Source: CAD feature listing. Evaluate the final solid. Frame: model axes, mm. Face numbers are marked on the shaded views. A direction names the side the tool comes from. Give positions to 0.01 mm unless a question says otherwise; leave off trailing zeros. Loops run counter-clockwise (first coordinate to the right, second up) from the corner with the lowest first, then second, coordinate; pieces in that order, holes last.
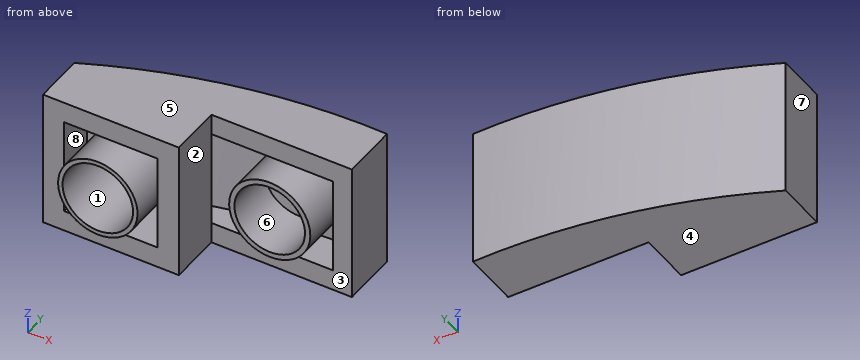
```python
from build123d import *

# Parameters (mm, degrees)
BOSS_EXTRUDE1_DEPTH      = 3.95
SHELL1_START             = -2.75
SHELL1_DEPTH             = 5.5
BOSS_EXTRUDE2_REACH      = 12.601
BOSS_EXTRUDE2_END_RADIUS = 32.700000868
BOSS_EXTRUDE2_START      = 1.2
SKETCH8_R                = 2.3
SKETCH8_R_2              = 2
BOSS_EXTRUDE3_REACH      = 13.983
BOSS_EXTRUDE3_END_RADIUS = 32.700000868
BOSS_EXTRUDE3_START      = 1.2
SKETCH9_R                = 2.25
SKETCH9_R_2              = 2
CUT_EXTRUDE5_DEPTH       = 13.479454835


# Read off the part's stored shape, not the designer's step: Shell1
with BuildPart() as part:
    # Sketch1 → Boss-Extrude1 (new, symmetric)
    with BuildSketch(Plane.XY):
        with BuildLine():
            Line((-7.9, -0.625209461), (-7.9, 2.229657062))
            ThreePointArc((-7.9, 2.229657062), (-0.19997769, 4.839494926), (7.9, 5.540892579))
            Line((7.9, 5.540892579), (7.9, 2.340892579))
            Line((7.9, 2.340892579), (-0.19997769, 2.340892579))
            Line((-0.19997769, 2.340892579), (-0.19997769, -0.625209461))
            Line((-0.19997769, -0.625209461), (-7.9, -0.625209461))
        make_face()
    extrude(amount=BOSS_EXTRUDE1_DEPTH, both=True)

    # Shell1 outline → Shell1 (cut)
    with BuildSketch(Plane.XY.offset(SHELL1_START)):
        with BuildLine():
            Line((-1.39997769, 2.340892579), (6.7, 2.340892579))
            Line((6.7, 2.340892579), (6.7, 4.360243445))
            ThreePointArc((6.7, 4.360243445), (-0.153454716, 3.622525068), (-6.7, 1.464559639))
            Line((-6.7, 1.464559639), (-6.7, -0.625209461))
            Line((-6.7, -0.625209461), (-1.39997769, -0.625209461))
            Line((-1.39997769, -0.625209461), (-1.39997769, 2.340892579))
        make_face()
    extrude(amount=SHELL1_DEPTH, mode=Mode.SUBTRACT)

    # Boss-Extrude2: up to this cylinder (the profile starts inside it)
    boss_extrude2_end = Plane(origin=(6.753451055, -28.339713738, 2.234946), z_dir=(0, 0, -1)) * Cylinder(BOSS_EXTRUDE2_END_RADIUS, 91.602001737, mode=Mode.PRIVATE)
    # Sketch8 → Boss-Extrude2 (add, up to the surface)
    with BuildSketch(Plane(origin=(0, 2.340892579, 0), x_dir=(-1, 0, 0), z_dir=(0, -1, 0)).offset(BOSS_EXTRUDE2_START), mode=Mode.PRIVATE) as boss_extrude2_sk1:
        with Locations(Location((-3.850011155, 0, 0), (0, 0, 90))):
            Circle(SKETCH8_R)
        with Locations(Location((-3.850011155, 0, 0), (0, 0, 90))):
            Circle(SKETCH8_R_2, mode=Mode.SUBTRACT)
    boss_extrude2_tool1 = extrude(boss_extrude2_sk1.sketch, amount=-BOSS_EXTRUDE2_REACH, mode=Mode.PRIVATE) & boss_extrude2_end
    add(boss_extrude2_tool1.solids().sort_by_distance((3.850011, 1.140893, 2.234946))[0])

    # Boss-Extrude3: up to this cylinder (the profile starts inside it)
    boss_extrude3_end = Plane(origin=(6.753451055, -28.339713738, 2.18636), z_dir=(0, 0, -1)) * Cylinder(BOSS_EXTRUDE3_END_RADIUS, 94.366001737, mode=Mode.PRIVATE)
    # Sketch9 → Boss-Extrude3 (add, up to the surface)
    with BuildSketch(Plane(origin=(0, -0.625209461, 0), x_dir=(-1, 0, 0), z_dir=(0, -1, 0)).offset(BOSS_EXTRUDE3_START), mode=Mode.PRIVATE) as boss_extrude3_sk1:
        with Locations(Location((4.049988845, 0, 0), (0, 0, 90))):
            Circle(SKETCH9_R)
        with Locations(Location((4.049988845, 0, 0), (0, 0, 90))):
            Circle(SKETCH9_R_2, mode=Mode.SUBTRACT)
    boss_extrude3_tool1 = extrude(boss_extrude3_sk1.sketch, amount=-BOSS_EXTRUDE3_REACH, mode=Mode.PRIVATE) & boss_extrude3_end
    add(boss_extrude3_tool1.solids().sort_by_distance((-4.049989, -1.825209, 2.18636))[0])

    # Sketch10 → Cut-Extrude5 (cut, through all)
    with BuildSketch(Plane(origin=(0, 0, -3.95), x_dir=(-1, 0, 0), z_dir=(0, 0, -1))):
        Polygon((-7.9, 2.340892579), (-7.760644151, 2.340892579), (-7.760644151, 5.545321616), (-7.9, 5.540892579), align=None)
    extrude(amount=-CUT_EXTRUDE5_DEPTH, mode=Mode.SUBTRACT)


with BuildPart() as cut_extrude5_kept_piece:
    # of the separate pieces the step leaves, the one the design keeps (cut_extrude5_pieces_kept)
    add(part.part.solids().sort_by_distance((-7.9, -0.625209461, -3.95))[0])


solid = cut_extrude5_kept_piece.part
```
(1) Section C-C, the plane x = 6.5. Return the cut outline in (y, z).
A:
outline: (2.34, -3.95) - (5.56, -3.95) - (5.56, 3.95) - (2.34, 3.95) - (2.34, 2.75) - (4.36, 2.75) - (4.36, -2.75) - (2.34, -2.75) - close
(2) Section A-A, the plane y = 0. Return the cut outline in (x, z).
A:
outline: (-7.9, -3.95) - (-0.2, -3.95) - (-0.2, 3.95) - (-7.9, 3.95) - close; circle Ø4.5 at (-4.05, 0); hole (-6.7, -2.75) - (-1.4, -2.75) - (-1.4, 2.75) - (-6.7, 2.75) - close; hole circle Ø4 at (-4.05, 0)
(3) Ray query, line 1 along X through (y, z) = (0.25, 0); line 2 along X through (y, z) = (1, 1.25); line 3 along X through (y, z) = (1.8, 0). Return the intervals inside material, ascending.
A:
line 1: x = -7.9 to -6.7, -6.3 to -6.05, -2.05 to -1.8, -1.4 to -0.2
line 2: x = -7.9 to -6.7, -5.92 to -5.61, -2.49 to -2.18, -1.4 to -0.2
line 3: x = -7.9 to -5.93, -2.05 to -1.8, -1.4 to -0.2, 1.55 to 1.85, 5.85 to 6.15
(4) Mould query, pull axis Z, two halves, no side actions, for the marked faces 5, 6, 7 and 8. Classes: pulls with the +Z half, pulls with the -Z half, needs draft (parallel to the pull), parting line crosses it, or undercut.
A:
face 5: pulls with the +Z half
face 6: undercut
face 7: needs draft
face 8: undercut
(5) Section D-D, the plane z = 3. Return the cut outline in (x, y).
A:
outline: (-7.9, -0.63) - (-0.2, -0.63) - (-0.2, 2.34) - (7.76, 2.34) - (7.76, 5.55) arc R33.9 ccw to (-7.9, 2.23) - close
(6) Section B-B, the plane z = 1.5. Return the cut outline in (x, y), then the cut area to 3 significant figures.
A:
outline: (-7.9, -0.63) - (-6.7, -0.63) - (-6.7, 1.46) arc R32.7 cw to (-5.73, 1.88) - (-5.73, -1.83) - (-5.37, -1.83) - (-5.37, 2.03) arc R32.7 cw to (-2.73, 2.96) - (-2.73, -1.83) - (-2.37, -1.83) - (-2.37, 3.06) arc R32.7 cw to (2.11, 4.03) - (2.11, 1.14) - (2.53, 1.14) - (2.53, 4.09) arc R32.7 cw to (5.17, 4.32) - (5.17, 1.14) - (5.59, 1.14) - (5.59, 4.34) arc R32.7 cw to (6.7, 4.36) - (6.7, 2.34) - (7.76, 2.34) - (7.76, 5.55) arc R33.9 ccw to (-7.9, 2.23) - close; (-1.4, -0.63) - (-0.2, -0.63) - (-0.2, 2.34) - (-1.4, 2.34) - close
area: 32.9 mm2
(7) First-contact query: pin 1 (1.5 mm diameter, centred on y = 0.5, z = -1.5, fed in from +X); pin 2 (3 mm diameter, centred on x = 3, y = 0.5, fed in from +Z); pin 3 (3 mm diameter, centred on x = 3.85, z = 0, fed in from +Y). Flat tips, straight axial feed; report the tip coordinate or a pass-through.
A:
pin 1: stops at x = 5.86
pin 2: stops at z = 2.3
pin 3: stops at y = 5.53
(8) Reachability of the marked faces 1, 2, 3 and 4 from +Z, -Z, +X, -X, +Y, -Y: full face, straight path, thin tool, end or side. Return the list, or none.
A:
face 1: -Y
face 2: +Z, -Z, -Y
face 3: +X, -Y
face 4: -Z, +X, -X, +Y, -Y
